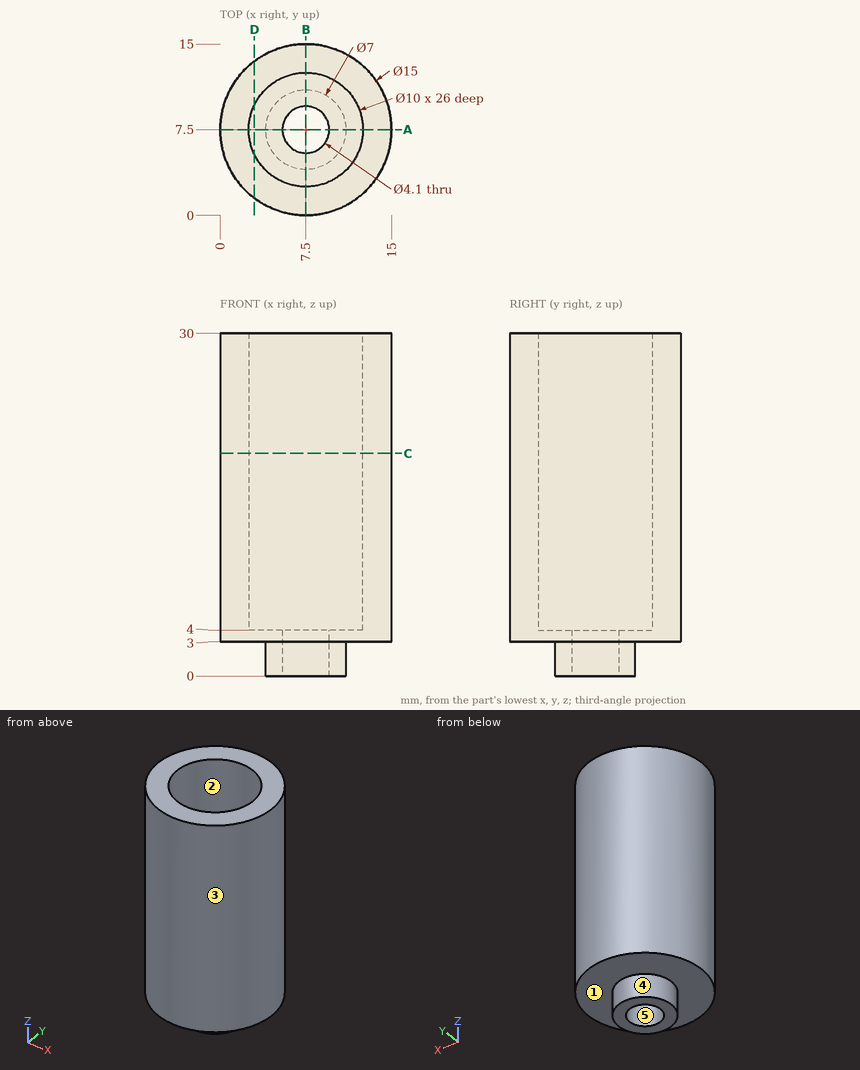
Source: three-view drawing plus pictorial views. Frame: mm from the lowest corner of the part. A direction names the side the tool comes from. Round coordinates to 2 decimals unless told otherwise and drop trailing zeros. Loops run counter-clockwise (first coordinate to the right, second up) from the corner with the lowest first, then second, coordinate; pieces in that order, holes last.
1. Access query for the marked faces 4 and 5. Directions: +Z, -Z, +X, -X, +Y, -Y. A direction counts if a zero-diameter tool reaches every point of the face in a straight line with its end or side. Return the directions, or none.
2. Section query C-C on z = 19.5. Output: boundary loops of the cut face in (x, y), and give its area (3 significant figures).
3. Section query A-A on y = 7.5. Output: boundary loops of the cut face in (x, z).
4. Mould query, pull axis Y, two halves, no side actions, for the marked faces 1, 2 and 3. Classes: released by +Y, released by -Y, zero draft, split by the parting line, or undercut.
5. Section query D-D on x = 3. Output: boundary loops of the cut face in (y, z), and give its area (3 significant figures).
6. Contact query for flat-ended pins moving along their axis: pin 1 (1.5 mm diameter, centred on x = 6, y = 13, fed in from -Z); pin 2 (3.5 mm diameter, centred on x = 7.5, y = 7.5, fed in from -Z); pin 3 (3 mm diameter, centred on x = 6, y = 9, fed in from +Z); pin 4 (2 mm diameter, centred on y = 2, z = 3.5, fed in from -X). Output: stop coordinate, or through.
7. Ray query, L1, parallel to Y at x = 7.5, z = 1.45; L2, parallel to Y at x = 7.5, z = 14.25. Return the intervals inside material, ascending.
Answers below:
1. face 4: -Z
1. face 5: +Z, -Z
2. outline: circle Ø15 at (7.5, 7.5); hole circle Ø10 at (7.5, 7.5)
2. area: 98.2 mm2
3. outline: (0, 3) - (4, 3) - (4, 0) - (5.45, 0) - (5.45, 4) - (2.5, 4) - (2.5, 30) - (0, 30) - close; (9.55, 0) - (11, 0) - (11, 3) - (15, 3) - (15, 30) - (12.5, 30) - (12.5, 4) - (9.55, 4) - close
4. face 1: zero draft
4. face 2: undercut
4. face 3: split by the parting line
5. outline: (1.5, 3) - (13.5, 3) - (13.5, 30) - (9.68, 30) - (9.68, 4) - (5.32, 4) - (5.32, 30) - (1.5, 30) - close
5. area: 211 mm2
6. pin 1: stops at z = 3
6. pin 2: passes through
6. pin 3: stops at z = 4
6. pin 4: stops at x = 1.5
7. L1: y = 4 to 5.45, 9.55 to 11
7. L2: y = 0 to 2.5, 12.5 to 15
